Geometry: final body of the model. Coordinates: model frame, mm. A direction names the side the tool comes from. Round coordinates to 2 decimals unless told otherwise and drop trailing zeros. Order: outer loops, then holes, each group sorted by start corner. A loop starts at its lowest first (then second) coordinate and runs counter-clockwise, first axis right, second up. Notation, with made-up numbers: (39, 81.5) -> (69, 81.5) arc R22 ccw to (69, 92.5) -> close; hole circle Ø4 at (-27, -27). An arc over 180 degrees is marked (long way). Put each result on its own line as item: value.
Autodesk Inventor part; units mm, degrees
ref_plane "YZ Plane" through (0, 0, 0) normal (1, 0, 0) x (0, 1, 0)
ref_plane "XZ Plane" through (0, 0, 0) normal (0, 1, 0) x (-1, 0, 0)
ref_plane "XY Plane" through (0, 0, 0) normal (0, 0, 1) x (1, 0, 0)
sketch "Sketch1" plane through (0, 0, 0) normal (0, 1, 0) x (-1, 0, 0)
  line L0 (0, 0) -> (85, 0)
  line L1 (85, 0) -> (85, -85)
  line L2 (85, -85) -> (0, -85)
  line L3 (0, -85) -> (0, 0)
  dimension "d0" = 85
  dimension "d1" = 85
extrude "Extrusion1" add sketch "Sketch1" along normal blind 6
fillet "Fillet1" radius 10 4 edges at (-85, 3, 0) (0, 3, 0) (0, 3, -85) (-85, 3, -85)
sketch "Sketch2" plane through (0, 6, 0) normal (0, 1, 0) x (1, 0, 0)
  line L0 (-75, 0) -> (-10, 0)
  line L1 (-57, 6.8542) -> (-35, 6.8542)
  line L2 (-35, 6.8542) -> (-35, 11.8542)
  line L3 (-35, 11.8542) -> (-35, 12.8542)
  line L4 (-35, 12.8542) -> (-57, 12.8542)
  line L5 (-57, 12.8542) -> (-57, 6.8542)
  point P0 (0, 0)
extrude "Extrusion2" add sketch "Sketch2" along normal blind 100
sketch "Sketch3" plane through (-57, 6, -6.8542) normal (0, 0, 1) x (1, 0, 0)
  line L0 (22, 100) -> (0, 100)
  line L1 (0, 100) -> (22, 100)
  line L2 (22, 100) -> (22, 92.8)
  line L3 (22, 0) -> (22, 100)
  line L4 (0, 0) -> (0, 100)
  line L5 (0, 100) -> (22, 91.9927)
  line L6 (0, 100) -> (23.4119, 100) construction
  line L7 (22, 91.9927) -> (22, 100)
  point P0 (57, -6)
  dimension "d12" = 7.2
  dimension "d13" = 20
extrude "Extrusion3" cut sketch "Sketch3" against normal blind 10
fillet "Fillet2" radius 3.5 2 edges at (-57, 106, -9.8542) (-35, 97.9927, -9.8542)
sketch "Sketch4" plane through (0, 6, 0) normal (0, 1, 0) x (1, 0, 0)
  point P0 (0, 0)
sketch "Sketch5" plane through (0, 6, 0) normal (0, 1, 0) x (1, 0, 0)
  line L0 (-57, 6.8542) -> (-57, 12.8542)
  line L1 (-57, 9.8542) -> (-55.64, 9.8542)
  circle A0 centre (-55.64, 9.8542) radius 1.36
  point P0 (0, 0)
  dimension "d19" = 2.72
extrude "Extrusion4" add sketch "Sketch5" along normal blind 100
sketch "Sketch6" plane through (-55.64, 106, -9.8542) normal (0, 1, 0) x (1, 0, 0)
  circle A0 centre (0, 0) radius 1.36
  point P0 (55.64, -9.8542)
extrude "Extrusion5" cut sketch "Sketch6" against normal blind 100
sketch "Sketch7" plane through (-57, 6, -6.8542) normal (-1, 0, 0) x (0, 0, 1)
  line L0 (-4.36, 97.771) -> (-4.36, 0)
  line L1 (-4.36, 97.771) -> (-1.64, 97.771)
  line L2 (-1.64, 97.771) -> (-1.64, 0)
  line L3 (-4.36, 97.771) -> (-4.36, 0)
  line L4 (-4.36, 0) -> (-1.64, 0)
  line L5 (-3.1458, 0) -> (6.8542, 0)
  line L6 (-1.64, 0) -> (-1.64, 97.771)
  line L7 (0, 98.5015) -> (0, 95.0015)
  point P0 (6.8542, -6)
  point P1 (0, 98.2904)
extrude "Extrusion6" cut sketch "Sketch7" against normal blind 1.36
sketch "Sketch8" plane through (-57, 6, -6.8542) normal (0, 0, 1) x (1, 0, 0)
  point P0 (57, -6)
sketch "Sketch9" plane through (-57, 6, -6.8542) normal (0, 0, 1) x (1, 0, 0)
  line L0 (0, 0) -> (0, 95.0015)
  line L1 (1.36, 0) -> (1.36, 97.771)
  line L2 (0, 0) -> (1.36, 0)
  line L3 (1.36, 0) -> (1.36, 3.2)
  line L4 (1.36, 3.2) -> (0, 3.2)
  line L5 (0, 3.2) -> (0, 0)
  line L6 (1.36, 0) -> (0, 0)
  line L7 (47, 0) -> (-18, 0)
  point P0 (57, -6)
  dimension "d26" = 3.2
extrude "Extrusion7" cut sketch "Sketch9" against normal blind 2
sketch "Sketch10" plane through (-35, 6, -6.8542) normal (0, 0, 1) x (1, 0, 0)
  line L0 (-20.64, 3.2) -> (-22, 3.2)
  line L1 (-20.64, 3.2) -> (-19.28, 3.2)
  line L2 (-19.28, 3.2) -> (-19.28, 0)
  line L3 (-19.28, 98.4135) -> (-19.28, 0)
  line L4 (25, 0) -> (-40, 0)
  line L5 (-20.64, 0) -> (-19.28, 0)
  line L6 (-20.64, 0) -> (-20.64, 97.771)
  line L7 (-20.64, 0) -> (-20.64, 3.2)
  point P0 (35, -6)
  dimension "d29" = 1.36
extrude "Extrusion8" cut sketch "Sketch10" against normal blind 3
properties part number "NewBase"
1. Contact query for flat-ended pins moving along their axis: P1, Ø2, axis at x = -55.5, y = 15.5, coming from the -Z side; P2, Ø0.9, axis at y = 8, z = -8.5, coming from the -X side; P3, Ø5, axis at y = 39.5, z = -10, coming from the +X side. Output: stop coordinate, or through.
Ans:
P1: z = -12.85
P2: x = -54.28
P3: x = -35
2. Draft query along Y for faces 4 (the face through (-42, 0, -42)), 5 (the face through (-56, 9.2, -8)), 6 (the face through (-46, 55, -12.854)). Return one class per face: +Y half, -Y half, draft (parallel to the pull), parting line (faces both ways), or undercut.
Ans:
face 4: -Y half
face 5: undercut
face 6: draft
3. Cut plane B-B on z = -43. Return loops of the section in (x, y), and give its area (3 significant figures).
Ans:
outline: (-85, 0) -> (0, 0) -> (0, 6) -> (-85, 6) -> close
area: 510 mm²
4. Cut plane A-A on y = 84. Return loops of the section in (x, z), and give its area (3 significant figures).
Ans:
outline: (-57, -12.85) -> (-35, -12.85) -> (-35, -6.85) -> (-57, -6.85) -> (-57, -8.49) -> (-55.64, -8.49) arc R1.36 cw to (-55.64, -11.21) -> (-57, -11.21) -> close
area: 125 mm²
5. Cut plane C-C on x = -60. Return loops of the section in (y, z), and give its area (3 significant figures).
Ans:
outline: (0, -85) -> (6, -85) -> (6, 0) -> (0, 0) -> close
area: 510 mm²
6. Material intervals for probe 1 along Y at (x, z) = (-41, -53); probe 2 along X at (y, z) = (83, -7); probe 3 along Z at (x, y) = (-44, 54), sorted ascending.
Ans:
probe 1: 0 to 6
probe 2: -57 to -35
probe 3: -12.85 to -6.85
7. Set-up query: faces 1 (the face through (-54.28, 8, -8)), 2 (the face through (-46, 55, -6.854)), 3 (the face through (-54.28, 55.9, -9.82)). Return all of +Z, -Z, +X, -X, +Y, -Y with unobstructed straight access to the full face (end or side cutting, diameter ignored); none if empty.
Ans:
face 1: +Z, -X
face 2: +Z, +X, -X, +Y
face 3: -X, +Y
